Verification items for this drawing (mm, ordinates from the low corner). Give positions to 0.01 mm unless a question says otherwise; leave off trailing zeros. Loops run counter-clockwise (first coordinate to the right, second up) from the corner with the lowest first, then second, coordinate; pieces in that order, holes last. Notation, with made-up numbers: M 57.25,75 L 99.25,75 A8 cw 99.25,82 Z; hole C 70,72 d6. An arc over 180 degrees is marked long. Use one line per item in the form item = value.
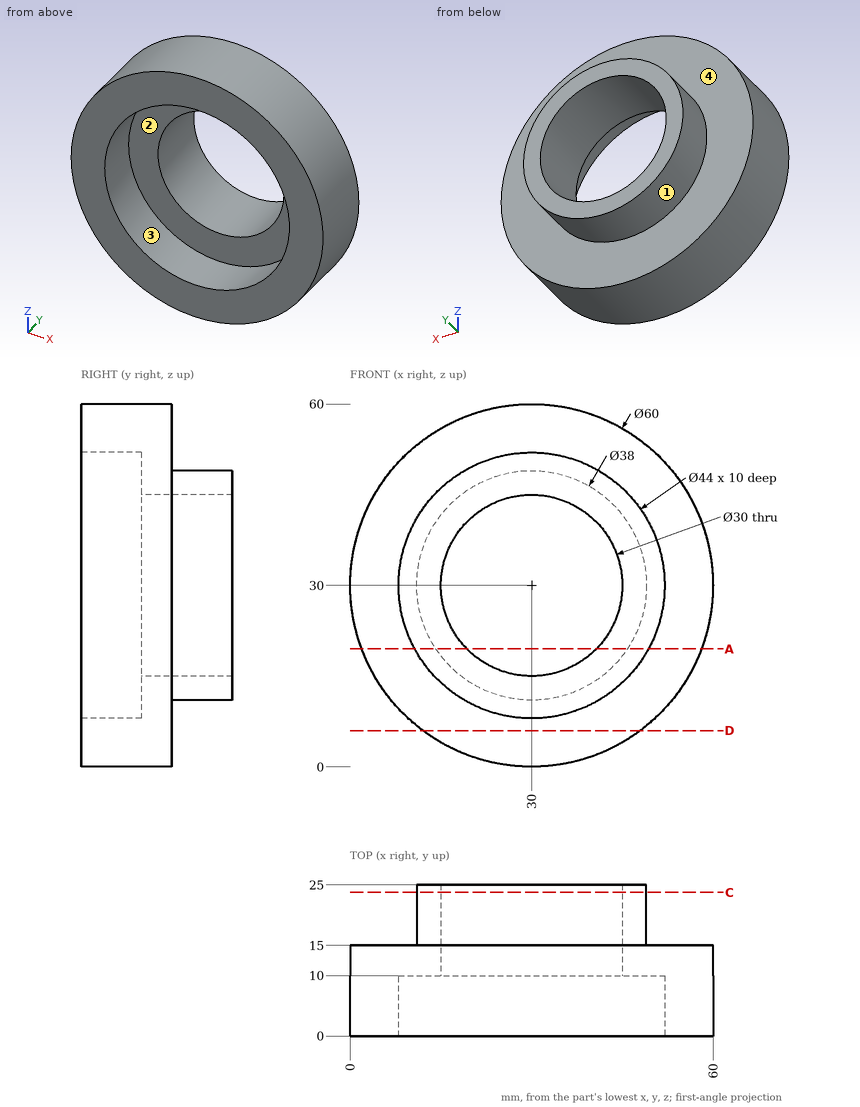
1) Section check C-C (y = 23.75). Record the cut outline in (x, z), then the cut area to 3 significant figures.
Evaluation:
outline = C 30,30 d38; hole C 30,30 d30
area = 427 mm^2
2) Section check A-A (z = 19.5). Record the cut outline in (x, y).
Evaluation:
outline = M 1.9,0 L 10.67,0 L 10.67,10 L 19.29,10 L 19.29,25 L 14.16,25 L 14.16,15 L 1.9,15 Z; M 40.71,10 L 49.33,10 L 49.33,0 L 58.1,0 L 58.1,15 L 45.84,15 L 45.84,25 L 40.71,25 Z
3) Depth check by flat-ended pin: pin 1 Ø1.5 at (x, y) = (30.5, 17) entering from -Z; pin 2 Ø5 at (x, y) = (7, 14) entering from +Z; pin 3 Ø1 at (y, z) = (12.5, 23) entering from -X; pin 4 Ø24 at (x, z) = (30, 30) entering from +Y. Enter the tip coordinate at first touch or a pass-through.
Evaluation:
pin_1 = 11
pin_2 = 51.9
pin_3 = 0.71
pin_4 = through
4) Release check for a two-part mould opening along Z. For the marked faces 1, 2, 3 and 4 record: pulls with the +Z half, pulls with the -Z half, needs draft (parallel to the pull), parting line crosses it, or undercut.
Evaluation:
face_1 = parting line crosses it
face_2 = undercut
face_3 = undercut
face_4 = needs draft
5) Scan lines: line 1 (X direction, y = 20.5, z = 30); line 2 (Z direction, x = 30, y = 4.75). Record each from-to range of solid material in increasing order.
Evaluation:
line_1 = 11 to 15, 45 to 49
line_2 = 0 to 8, 52 to 60
6) Section check D-D (z = 6). Record the cut outline in (x, y), then the cut area to 3 significant figures.
Evaluation:
outline = M 12,0 L 48,0 L 48,15 L 12,15 Z
area = 540 mm^2
